Here's how the part is built. I have some questions about the finished solid (model axes, mm). Give positions to 0.01 mm unless a question says otherwise; leave off trailing zeros. Order: outer loops, then holes, each group sorted by start corner. A loop starts at its lowest first (then second) coordinate and runs counter-clockwise, first axis right, second up. Notation, with made-up numbers: M 17,74.25 L 29,74.25 A14 cw 29,85.25 Z; hole C 85,46 d3. An arc over 180 degrees is marked long. Use one line per item in the form item = value.
Autodesk Inventor part; units mm, degrees
ref_plane "YZ Plane" through (0, 0, 0) normal (1, 0, 0) x (0, 1, 0)
ref_plane "XZ Plane" through (0, 0, 0) normal (0, 1, 0) x (-1, 0, 0)
ref_plane "XY Plane" through (0, 0, 0) normal (0, 0, 1) x (1, 0, 0)
sketch "Sketch1" plane through (0, 0, 0) normal (0, 0, 1) x (1, 0, 0)
  circle A0 centre (0, 0) radius 12.7
  circle A1 centre (0, 0) radius 3.302
  dimension "d0" = 25.4
  dimension "d1" = 6.604
extrude "Extrusion1" add sketch "Sketch1" along normal mid plane 120.65
fillet "Fillet1" radius 3 2 edges at (-12.7, 0, 60.325) (-12.7, 0, -60.325)
sketch "Sketch3" plane through (0, 0, 60.325) normal (0, 0, 1) x (1, 0, 0)
  line L0 (-31, 0) -> (39, 0)
  line L1 (39, 0) -> (17, 30)
  line L2 (17, 30) -> (-16, 29)
  line L3 (-16, 29) -> (-31, 0)
extrude "Extrusion2" cut sketch "Sketch3" against normal through all
properties part number "Wagon Hand Handle V03"
Q1. I want a section at B-B on x = 0. Write out the boundary of the cut face in (y, z) (3 decimals).
Found:
outline = M -12.7,-57.325 A3 ccw -9.7,-60.325 L -3.302,-60.325 L -3.302,60.325 L -9.7,60.325 A3 ccw -12.7,57.325 Z
Q2. I want a section at A-A on z = 11. Write out the boundary of the cut face in (x, y).
Found:
outline = M -12.7,0 A12.7 ccw 12.7,0 L 3.3,0 A3.3 cw -3.3,0 Z
Q3. I need wall thicknesses on L1, parallel to X at y = -1, z = -24; L2, parallel to Z at x = 4.75, y = -9.5; L3, parallel to X at y = -5.5, z = 9.5. Which ranges of each line are inside material? Lowest first, please.
Found:
L1 = -12.66 to -3.15, 3.15 to 12.66
L2 = -60.18 to 60.18
L3 = -11.45 to 11.45
Q4. I'm going to push flat-ended pins straight in: pin 1 Ø3 at (x, z) = (-4, -19) entering from -Y; pin 2 Ø3 at (x, z) = (5.5, -28) entering from -Y; pin 3 Ø1 at (y, z) = (-3.5, 29) entering from -X. Where does each tip first touch, or does it pass through?
Found:
pin_1 = -12.45
pin_2 = -12.05
pin_3 = -12.34
